Input: part model. Units: mm. Frame: model coordinates. A direction names the side the tool comes from. Coordinates: 2 decimals unless noted, no trailing zeros. Order: outer loops, then holes, each group sorted by start corner. A loop starts at its lowest first (then second) coordinate and runs counter-clockwise, first axis right, second up. Notation, with made-up numbers: (10, 77.5) -> (39, 77.5) arc R18 ccw to (39, 103.5) -> close; hole circle Ø3 at (41.5, 35.5). An arc over 180 degrees is marked (long way). Use one line per item in the form item = value. Start each with the question number.
1) Section query B-B on z = -11. Output: boundary loops of the cut face in (x, y) (3 decimals), then the cut area to 3 significant figures.
2) Draft query along Z for faces 1 (the flat face through (-2, -30.619, -30)), 2 (the cylindrical face through (-1.61, -25.253, -22.247)), 3 (the cylindrical face through (-1.565, -28.861, -47.514)). Return one class per face: pulls with the +Z half, pulls with the -Z half, needs draft (parallel to the pull), parting line crosses it, or undercut.
3) Section query C-C on y = -21. Output: boundary loops of the cut face in (x, z) (3 decimals).
4) Pin query (flat end, axial travel): pin 1 (1.4 mm diameter, centred on y = -25.4, z = -23.368, fed in from -X); pin 2 (6 mm diameter, centred on x = 12, z = -5.5, fed in from -Y); pin 3 (3 mm diameter, centred on y = -25.4, z = -17.018, fed in from +X); pin 4 (1 mm diameter, centred on x = -1.5, z = -38.5, fed in from +Y). Return the tip coordinate at first contact, or that it passes through.
5) Access query for faces 4 (the cylindrical face through (26.145, 1.565, -19.59)), 5 (the flat face through (-2, -21.729, -36)), 6 (the flat face through (22, 0, -13)). Directions: +Z, -Z, +X, -X, +Y, -Y. A direction counts if a zero-diameter tool reaches every point of the face in a straight line with its end or side. Return the directions, or none.
6) Ray query, line 1 along X through (y, z) = (-6, -4) (3 decimals); line 2 along Z through (x, y) = (-1.75, -25.4); line 3 along Z through (x, y) = (-1, -25). Return the intervals inside material, ascending.
7) Section query A-A on z = -19.05. Output: boundary loops of the cut face in (x, y) (3 decimals), then the cut area to 3 significant figures.
8) Section query D-D on x = 8. Output: boundary loops of the cut face in (y, z) (3 decimals), then the cut area to 3 significant figures.
from build123d import *

# Parameters (mm, degrees)
SKETCH1_R                  = 2.4892
BOSS_EXTRUDE1_DEPTH        = 3.175
SKETCHED_START             = -52
SKETCHED_BEND2_DEPTH       = 52
SKETCHED_START_2           = -25.4
SKETCHED_BEND2_2_DEPTH     = 12.7
SKETCHED_START_3           = -41.835294118
SKETCHED_BEND2_3_OUTLINE_W = 3.175
SKETCHED_BEND2_3_OUTLINE_H = 12.7
SKETCHED_BEND2_3_DEPTH     = 16.435294118
SKETCHED_BEND2_4_DEPTH     = 20.459192
SKETCHED_START_4           = -50.8
SKETCHED_BEND2_5_OUTLINE_W = 3.175
SKETCHED_BEND2_5_OUTLINE_H = 12.7
SKETCHED_BEND2_5_DEPTH     = 48.117252
SKETCHED_START_5           = -4.940808
SKETCHED_BEND2_6_DEPTH     = 4.940808
SKETCHED_START_6           = -3.175
SKETCHED_BEND2_7_DEPTH     = 3.175
SKETCH13_R                 = 1.1303
CUT_EXTRUDE2_DEPTH         = 75.121324278
FILLET1_R                  = 3.175
SKETCH14_W                 = 20.670157998
SKETCH14_H                 = 6.985
CUT_EXTRUDE3_DEPTH         = 71.21778451
FILLET2_R                  = 3.175


with BuildPart() as part:
    # Sketch1 → Boss-Extrude1 (new body)
    # profile 1 of 2: a face of its own
    with BuildSketch(Plane(origin=(0, 0, 0), x_dir=(1, 0, 0), z_dir=(0, 1, 0))):
        Polygon((6.35, 0), (25.4, 0), (28.575, 0), (41.275, 0), (41.275, 25.4), (27.523477182, 25.4), (14.823477182, 25.4), (6.35, 25.4), align=None)
        with Locations(Location((28.575, 6.35, 0), (0, 0, 270))):
            Circle(SKETCH1_R, mode=Mode.SUBTRACT)
        with Locations(Location((28.575, 19.05, 0), (0, 0, 270))):
            Circle(SKETCH1_R, mode=Mode.SUBTRACT)
    # profile 2 of 2: a face of its own
    with BuildSketch(Plane(origin=(0, 0, 0), x_dir=(1, 0, 0), z_dir=(0, 1, 0))):
        Polygon((-12.7, 0), (6.35, 0), (6.35, 25.4), (0, 25.4), (-19.05, 25.4), (-19.05, 41.835294118), (-23.415467049, 44.91680027), (-31.75, 50.8), (-31.75, 12.7), (-23.415467049, 7.143644699), align=None)
    extrude(amount=BOSS_EXTRUDE1_DEPTH)

    # Sketched Bend2: read off the stored shape, not the designer's step
    # Sketched Bend2 outline → Sketched Bend2 (cut)
    with BuildSketch(Plane.XY.offset(SKETCHED_START)):
        with BuildLine():
            ThreePointArc((-2.324261315, 0), (-1e-09, 2.324261314), (3.175, 3.175))
            Line((3.175, 3.175), (-31.75, 3.175))
            Line((-31.75, 3.175), (-31.75, 0))
            Line((-31.75, 0), (-2.324261315, 0))
        make_face()
    extrude(amount=SKETCHED_BEND2_DEPTH, mode=Mode.SUBTRACT)

    # Sketched Bend2 2 outline → Sketched Bend2 2 (add)
    with BuildSketch(Plane.XY.offset(SKETCHED_START_2)):
        with BuildLine():
            ThreePointArc((-2.324261315, 0), (-2.958628997, -1.531499064), (-3.175, -3.175))
            Line((-3.175, -3.175), (-3.175, -30.619082494))
            Line((-3.175, -30.619082494), (0, -30.619082494))
            Line((0, -30.619082494), (0, -3.175))
            ThreePointArc((0, -3.175), (0.92993597, -0.92993597), (3.175, 0))
            Line((3.175, 0), (-2.324261315, 0))
        make_face()
    extrude(amount=SKETCHED_BEND2_2_DEPTH)

    # Sketched Bend2 3 outline → Sketched Bend2 3 (add)
    with BuildSketch(Plane.XY.offset(SKETCHED_START_3)):
        with Locations((-1.5875, -24.269082494)):
            Rectangle(SKETCHED_BEND2_3_OUTLINE_W, SKETCHED_BEND2_3_OUTLINE_H)
    extrude(amount=SKETCHED_BEND2_3_DEPTH)

    # Sketched Bend2 4 outline → Sketched Bend2 4 (add)
    with BuildSketch(Plane.XY.offset(SKETCHED_START_2)):
        with BuildLine():
            ThreePointArc((-2.324261315, 0), (-2.958628997, -1.531499064), (-3.175, -3.175))
            Line((-3.175, -3.175), (-3.175, -17.919082494))
            Line((-3.175, -17.919082494), (0, -17.919082494))
            Line((0, -17.919082494), (0, -3.175))
            ThreePointArc((0, -3.175), (0.92993597, -0.92993597), (3.175, 0))
            Line((3.175, 0), (-2.324261315, 0))
        make_face()
    extrude(amount=SKETCHED_BEND2_4_DEPTH)

    # Sketched Bend2 5 outline → Sketched Bend2 5 (add)
    with BuildSketch(Plane.XY.offset(SKETCHED_START_4)):
        with Locations((-1.5875, -24.269082494)):
            Rectangle(SKETCHED_BEND2_5_OUTLINE_W, SKETCHED_BEND2_5_OUTLINE_H)
    extrude(amount=SKETCHED_BEND2_5_DEPTH)

    # Sketched Bend2 6 outline → Sketched Bend2 6 (add)
    with BuildSketch(Plane.XY.offset(SKETCHED_START_5)):
        with BuildLine():
            ThreePointArc((-2.324261315, 0), (-2.958628997, -1.531499064), (-3.175, -3.175))
            Line((-3.175, -3.175), (-3.175, -17.919082494))
            Line((-3.175, -17.919082494), (0, -17.919082494))
            Line((0, -17.919082494), (0, -3.175))
            ThreePointArc((0, -3.175), (0.92993597, -0.92993597), (3.175, 0))
            Line((3.175, 0), (-2.324261315, 0))
        make_face()
    extrude(amount=SKETCHED_BEND2_6_DEPTH)

    # Sketched Bend2 7 outline → Sketched Bend2 7 (cut)
    with BuildSketch(Plane.YZ.offset(SKETCHED_START_6)):
        Polygon((-30.619082494, -2.682748), (-30.619082494, -12.7), (-11.569082494, 0), (-17.919082494, 0), (-17.919082494, -2.682748), align=None)
        Polygon((-17.919082494, -41.835294118), (-30.619082494, -50.8), (-17.919082494, -50.8), align=None)
    extrude(amount=SKETCHED_BEND2_7_DEPTH, mode=Mode.SUBTRACT)

    # Sketch13 → Cut-Extrude2 (cut, through all)
    with BuildSketch(Plane.ZY.offset(3.175)):
        with Locations(Location((-17.018, -25.4, 0), (0, 0, 270))):
            Circle(SKETCH13_R)
        with Locations(Location((-23.368, -25.4, 0), (0, 0, 270))):
            Circle(SKETCH13_R)
        with Locations(Location((-29.718, -25.4, 0), (0, 0, 270))):
            Circle(SKETCH13_R)
        with Locations(Location((-36.068, -25.4, 0), (0, 0, 270))):
            Circle(SKETCH13_R)
        with Locations(Location((-42.418, -25.4, 0), (0, 0, 270))):
            Circle(SKETCH13_R)
    extrude(amount=-CUT_EXTRUDE2_DEPTH, mode=Mode.SUBTRACT)

    # Fillet1
    fillet1_edges = [part.edges().sort_by_distance(p)[0] for p in [
        (-1.5875, -17.919082494, -41.835294118),
        (-1.5875, -17.919082494, -25.4),
        (-1.5875, -11.569082494, 0),
        (-1.5875, -30.619082494, -12.7),
        (-1.5875, -30.619082494, -50.8),
        (41.275, 1.5875, -25.4),
        (41.275, 1.5875, 0),
    ]]
    fillet(fillet1_edges, radius=FILLET1_R)

    # Sketch14 → Cut-Extrude3 (cut, through all)
    with BuildSketch(Plane(origin=(0, 0, 0), x_dir=(0, 0, -1), z_dir=(1, 0, 0))):
        with Locations((35.735078999, -18.236582494)):
            Rectangle(SKETCH14_W, SKETCH14_H)
    extrude(amount=-CUT_EXTRUDE3_DEPTH, mode=Mode.SUBTRACT)

    # Fillet2
    fillet2_edges = [part.edges().sort_by_distance(p)[0] for p in [
        (-1.5875, -21.729082494, -44.524705882),
        (-1.5875, -21.729082494, -25.4),
    ]]
    fillet(fillet2_edges, radius=FILLET2_R)


solid = part.part
Answers below:
q1.outline = (-3.175, -28.069) -> (0, -28.069) -> (0, -3.175) arc R3.175 cw to (3.175, 0) -> (41.275, 0) -> (41.275, 3.175) -> (3.175, 3.175) arc R6.35 ccw to (-3.175, -3.175) -> close
q1.area = 224 mm^2
q2.face_1 = needs draft
q2.face_2 = undercut
q2.face_3 = pulls with the -Z half
q3.outline = (-3.175, -26.551) -> (0, -26.551) -> (0, -6.287) -> (-3.175, -6.287) -> close
q4.pin_1 = through
q4.pin_2 = 0
q4.pin_3 = 0
q4.pin_4 = -21.73
q5.face_4 = +Y, -Y
q5.face_5 = -Z, +X, -X, +Y
q5.face_6 = +Z, -Z, +X, -Y
q6.line_1 = -3.175 to 0
q6.line_2 = -47.12 to -43.55, -41.29 to -37.2, -34.94 to -30.85, -28.59 to -24.5, -22.24 to -18.15, -15.89 to -9.22
q6.line_3 = -46.83 to -43.48, -41.36 to -37.13, -35.01 to -30.78, -28.66 to -24.43, -22.31 to -18.08, -15.96 to -8.95
q7.outline = (-3.175, -30.619) -> (0, -30.619) -> (0, -3.175) arc R3.175 cw to (3.175, 0) -> (26.086, 0) -> (26.086, 3.175) -> (3.175, 3.175) arc R6.35 ccw to (-3.175, -3.175) -> close; (31.064, 0) -> (41.275, 0) -> (41.275, 3.175) -> (31.064, 3.175) -> close
q7.area = 216 mm^2
q8.outline = (0, -25.4) -> (3.175, -25.4) -> (3.175, 0) -> (0, 0) -> close
q8.area = 80.6 mm^2
